from build123d import *

# Parameters (mm, degrees)
SKETCH1_W                       = 260
SKETCH1_H                       = 350
BOSS_EXTRUDE1_DEPTH             = 58
FILLET1_R                       = 54
SKIZZE1_W                       = 260
SKIZZE1_H                       = 350
SKIZZE1_W_2                     = 248
SKIZZE1_H_2                     = 338
SCHNITT_LINEAR_AUSTRAGEN1_DEPTH = 4
M4_TAPPED_HOLE1_AT_2_COUNT      = 2
M4_TAPPED_HOLE1_AT_2_PITCH      = 70
M4_TAPPED_HOLE1_AT_3_COUNT      = 2
M4_TAPPED_HOLE1_AT_3_PITCH      = 60.638271743
M4_TAPPED_HOLE1_AT_4_COUNT      = 2
M4_TAPPED_HOLE1_AT_4_PITCH      = 129.757466067
SKETCH2_W                       = 260
SKETCH2_H                       = 350
CUT_EXTRUDE1_DEPTH              = 225.590738901
M8_TAPPED_HOLE1_D               = 6.8
CIRPATTERN1_COUNT               = 2


with BuildPart() as part:
    # Sketch1 → Boss-Extrude1 (new body)
    with BuildSketch(Plane.XY):
        Rectangle(SKETCH1_W, SKETCH1_H)
    extrude(amount=BOSS_EXTRUDE1_DEPTH)

    # Fillet1
    fillet1_edges = [part.edges().sort_by_distance(p)[0] for p in [
        (130, 0, 58),
        (0, 175, 58),
        (-130, 0, 58),
        (0, -175, 58),
    ]]
    fillet(fillet1_edges, radius=FILLET1_R)

    # Skizze1 → Schnitt-Linear austragen1 (cut)
    with BuildSketch(Plane(origin=(0, 0, 0), x_dir=(-1, 0, 0), z_dir=(0, 0, -1))):
        Rectangle(SKIZZE1_W, SKIZZE1_H)
        Rectangle(SKIZZE1_W_2, SKIZZE1_H_2, mode=Mode.SUBTRACT)
    extrude(amount=-SCHNITT_LINEAR_AUSTRAGEN1_DEPTH, mode=Mode.SUBTRACT)

    # Skizze2 → M4 Tapped Hole1 (revolve, cut)
    with BuildSketch(Plane(origin=(105, 164, 0), x_dir=(0, 1, 0), z_dir=(1, 0, 0))):
        Polygon((0, 0), (0, 12.491420021), (1.65, 11.5), (1.65, 0), align=None)
    m4_tapped_hole1 = revolve(axis=Axis((105, 164, -6.35), (0, 0, 1)), mode=Mode.SUBTRACT)

    # M4 Tapped Hole1 at 2: M4 Tapped Hole1 ×2
    with Locations(*[(-i * M4_TAPPED_HOLE1_AT_2_PITCH, 0, 0) for i in range(1, M4_TAPPED_HOLE1_AT_2_COUNT)]):
        add(m4_tapped_hole1, mode=Mode.SUBTRACT)

    # M4 Tapped Hole1 at 3: M4 Tapped Hole1 ×2
    with Locations(*[Vector(0.23087729246792194, -0.9729828754005292, 0) * (i * M4_TAPPED_HOLE1_AT_3_PITCH) for i in range(1, M4_TAPPED_HOLE1_AT_3_COUNT)]):
        add(m4_tapped_hole1, mode=Mode.SUBTRACT)

    # M4 Tapped Hole1 at 4: M4 Tapped Hole1 ×2
    with Locations(*[Vector(0.10789359891495286, -0.9941624471449217, 0) * (i * M4_TAPPED_HOLE1_AT_4_PITCH) for i in range(1, M4_TAPPED_HOLE1_AT_4_COUNT)]):
        add(m4_tapped_hole1, mode=Mode.SUBTRACT)

    # Spiegeln1: M4 Tapped Hole1 across plane
    add(m4_tapped_hole1.mirror(Plane.ZX), mode=Mode.SUBTRACT)

    # Spiegeln1 copy 1 sketch → Spiegeln1 copy 1 (revolve, cut)
    with BuildSketch(Plane(origin=(35, -164, 0), x_dir=(0, -1, 0), z_dir=(1, 0, 0))):
        Polygon((0, 0), (0, -12.491420021), (1.65, -11.5), (1.65, 0), align=None)
    revolve(axis=Axis((35, -164, -6.35), (0, 0, -1)), mode=Mode.SUBTRACT)

    # Spiegeln1 copy 2 sketch → Spiegeln1 copy 2 (revolve, cut)
    with BuildSketch(Plane(origin=(119, -105, 0), x_dir=(0, -1, 0), z_dir=(1, 0, 0))):
        Polygon((0, 0), (0, -12.491420021), (1.65, -11.5), (1.65, 0), align=None)
    revolve(axis=Axis((119, -105, -6.35), (0, 0, -1)), mode=Mode.SUBTRACT)

    # Spiegeln1 copy 3 sketch → Spiegeln1 copy 3 (revolve, cut)
    with BuildSketch(Plane(origin=(119, -35, 0), x_dir=(0, -1, 0), z_dir=(1, 0, 0))):
        Polygon((0, 0), (0, -12.491420021), (1.65, -11.5), (1.65, 0), align=None)
    revolve(axis=Axis((119, -35, -6.35), (0, 0, -1)), mode=Mode.SUBTRACT)

    # Spiegeln2: M4 Tapped Hole1 across plane
    add(m4_tapped_hole1.mirror(Plane(origin=(0, 0, 0), x_dir=(0, 0, 1), z_dir=(1, 0, 0))), mode=Mode.SUBTRACT)

    # Spiegeln2 copy 1 sketch → Spiegeln2 copy 1 (revolve, cut)
    with BuildSketch(Plane(origin=(-35, 164, 0), x_dir=(0, 1, 0), z_dir=(-1, 0, 0))):
        Polygon((0, 0), (0, -12.491420021), (1.65, -11.5), (1.65, 0), align=None)
    revolve(axis=Axis((-35, 164, -6.35), (0, 0, -1)), mode=Mode.SUBTRACT)

    # Spiegeln2 copy 2 sketch → Spiegeln2 copy 2 (revolve, cut)
    with BuildSketch(Plane(origin=(-119, 105, 0), x_dir=(0, 1, 0), z_dir=(-1, 0, 0))):
        Polygon((0, 0), (0, -12.491420021), (1.65, -11.5), (1.65, 0), align=None)
    revolve(axis=Axis((-119, 105, -6.35), (0, 0, -1)), mode=Mode.SUBTRACT)

    # Spiegeln2 copy 3 sketch → Spiegeln2 copy 3 (revolve, cut)
    with BuildSketch(Plane(origin=(-119, 35, 0), x_dir=(0, 1, 0), z_dir=(-1, 0, 0))):
        Polygon((0, 0), (0, -12.491420021), (1.65, -11.5), (1.65, 0), align=None)
    revolve(axis=Axis((-119, 35, -6.35), (0, 0, -1)), mode=Mode.SUBTRACT)

    # Spiegeln2 copy 4 sketch → Spiegeln2 copy 4 (revolve, cut)
    with BuildSketch(Plane(origin=(-105, -164, 0), x_dir=(0, -1, 0), z_dir=(-1, 0, 0))):
        Polygon((0, 0), (0, 12.491420021), (1.65, 11.5), (1.65, 0), align=None)
    revolve(axis=Axis((-105, -164, -6.35), (0, 0, 1)), mode=Mode.SUBTRACT)

    # Spiegeln2 copy 5 sketch → Spiegeln2 copy 5 (revolve, cut)
    with BuildSketch(Plane(origin=(-35, -164, 0), x_dir=(0, -1, 0), z_dir=(-1, 0, 0))):
        Polygon((0, 0), (0, 12.491420021), (1.65, 11.5), (1.65, 0), align=None)
    revolve(axis=Axis((-35, -164, -6.35), (0, 0, 1)), mode=Mode.SUBTRACT)

    # Spiegeln2 copy 6 sketch → Spiegeln2 copy 6 (revolve, cut)
    with BuildSketch(Plane(origin=(-119, -105, 0), x_dir=(0, -1, 0), z_dir=(-1, 0, 0))):
        Polygon((0, 0), (0, 12.491420021), (1.65, 11.5), (1.65, 0), align=None)
    revolve(axis=Axis((-119, -105, -6.35), (0, 0, 1)), mode=Mode.SUBTRACT)

    # Spiegeln2 copy 7 sketch → Spiegeln2 copy 7 (revolve, cut)
    with BuildSketch(Plane(origin=(-119, -35, 0), x_dir=(0, -1, 0), z_dir=(-1, 0, 0))):
        Polygon((0, 0), (0, 12.491420021), (1.65, 11.5), (1.65, 0), align=None)
    revolve(axis=Axis((-119, -35, -6.35), (0, 0, 1)), mode=Mode.SUBTRACT)

    # Sketch2 → Cut-Extrude1 (cut, through all)
    with BuildSketch(Plane(origin=(0, 0, 4), x_dir=(-1, 0, 0), z_dir=(0, 0, -1))):
        Rectangle(SKETCH2_W, SKETCH2_H)
    extrude(amount=-CUT_EXTRUDE1_DEPTH, mode=Mode.SUBTRACT)

    # M8 Tapped Hole1 (through all)
    with Locations(Plane(origin=(0, 0, 0), x_dir=(-1, 0, 0), z_dir=(0, 0, -1))):
        with Locations((-82.5, -55)):
            m8_tapped_hole1 = Hole(M8_TAPPED_HOLE1_D / 2)

    # CirPattern1: M8 Tapped Hole1 ×2 about axis
    cirpattern1_axis = Axis((0, 0, 0), (0, 0, 1))
    for i in range(1, CIRPATTERN1_COUNT):
        add(m8_tapped_hole1.rotate(cirpattern1_axis, i * 360 / CIRPATTERN1_COUNT), mode=Mode.SUBTRACT)


solid = part.part
The model under review builds one solid part; all positions refer to its coordinate system, in mm. Give positions to 0.01 mm unless a question says otherwise; leave off trailing zeros. Order: outer loops, then holes, each group sorted by start corner. A loop starts at its lowest first (then second) coordinate and runs counter-clockwise, first axis right, second up. Notation, with made-up numbers: M -16,-6.5 L -9,-6.5 A21 ccw -9,26.5 Z; hole C -32.5,60.5 d11. An arc over 180 degrees is marked long. Answer in a Markdown table with one row per item. Add a question column.
1. Add section A-A on x = -82.5. State the section outline as (y, z) points.
2. Add section B-B on y = -55. State the section outline as (x, z) points.
3. For pin 1 Ø4 at (x, y) = (119, -35) entering from +Z; pin 2 Ø3 at (x, y) = (35, 164) entering from -Z, all flat-tipped, find the tip position at first contact; note any pin that passes through.
4. Mouldability with a two-part tool opening along X and no side actions: class faces 1 (the cylindrical face through (-79.994, 52.702, 2.028)), 2 (the flat face through (-2, 2, 0)) as released by +X, released by -X, zero draft, split by the parting line, or undercut.
5. To check wall thickness, follow line 1 along X through (y, z) = (164, 2.95); line 2 along X through (y, z) = (-105, 3.15); line 3 along Y through (x, z) = (35, 1.4). State the ranges of each line that lie inside material, in increasing order.
The answers:
| question | item | result |
|---|---|---|
| 1 | outline | M -169,0 L 51.6,0 L 51.6,4 L -169,4 Z; M 58.4,0 L 169,0 L 169,4 L 58.4,4 Z |
| 2 | outline | M -124,0 L 79.1,0 L 79.1,4 L -124,4 Z; M 85.9,0 L 124,0 L 124,4 L 85.9,4 Z |
| 3 | pin 1 | z = 4 |
| 3 | pin 2 | through |
| 4 | face 1 | undercut |
| 4 | face 2 | zero draft |
| 5 | line 1 | -124 to -106.65, -103.35 to -36.65, -33.35 to 33.35, 36.65 to 103.35, 106.65 to 124 |
| 5 | line 2 | -124 to -120.65, -117.35 to 117.35, 120.65 to 124 |
| 5 | line 3 | -169 to -165.65, -162.35 to 162.35, 165.65 to 169 |
